```python
from build123d import *

# Parameters (mm, degrees)
SKETCH3_R                = 15
BOSS_EXTRUDE2_DEPTH      = 40
BOSS_EXTRUDE3_DEPTH      = 30
BOSS_EXTRUDE3_DEPTH_BACK = 30
SKETCH4_R                = 10
SKETCH5_OUTSIDE_W        = 57.62
SKETCH5_OUTSIDE_H        = 47.62
SKETCH5_OUTSIDE_R        = 10
SKETCH5_OUTSIDE_R_2      = 6
CUT_EXTRUDE2_DEPTH       = 10


with BuildPart() as part:
    # Sketch3 → Boss-Extrude2 (new body)
    with BuildSketch(Plane.XY):
        Circle(SKETCH3_R)
    extrude(amount=BOSS_EXTRUDE2_DEPTH)

    # Sketch4 → Boss-Extrude3 (add, two sides: drawn at the far end of the back side and taken through both)
    with BuildSketch(Plane(origin=(0, 0, 0), x_dir=(0, 0, -1), z_dir=(1, 0, 0)).offset(-BOSS_EXTRUDE3_DEPTH_BACK)):
        with Locations((-20, 0)):
            Circle(SKETCH4_R)
    extrude(amount=BOSS_EXTRUDE3_DEPTH + BOSS_EXTRUDE3_DEPTH_BACK)

    # Sketch5 outside → Cut-Extrude2 (cut)
    # profile 1 of 2: a face of its own
    with BuildSketch(Plane(origin=(30, 0, 0), x_dir=(0, 0, -1), z_dir=(1, 0, 0))):
        with Locations((-20, 0)):
            Rectangle(SKETCH5_OUTSIDE_W, SKETCH5_OUTSIDE_H)
        with Locations((-20, 0)):
            Circle(SKETCH5_OUTSIDE_R, mode=Mode.SUBTRACT)
    # profile 2 of 2: a face of its own
    with BuildSketch(Plane(origin=(30, 0, 0), x_dir=(0, 0, -1), z_dir=(1, 0, 0))):
        with Locations((-20, 0)):
            Circle(SKETCH5_OUTSIDE_R_2)
    extrude(amount=-CUT_EXTRUDE2_DEPTH, mode=Mode.SUBTRACT)


solid = part.part
```
Input: part model. Units: mm. Frame: model coordinates. A direction names the side the tool comes from. Round coordinates to 2 decimals unless told otherwise and drop trailing zeros. Loops run counter-clockwise (first coordinate to the right, second up) from the corner with the lowest first, then second, coordinate; pieces in that order, holes last. Notation, with made-up numbers: (-5, 41.5) - (9, 41.5) arc R9 cw to (9, 52.5) - close; hole circle Ø8 at (30, -2). An arc over 180 degrees is marked (long way). One line per item, written item: value. Start each with the question number.
(1) Section D-D, the plane x = 17.5. Return loops of the section in (y, z), plus the area to 3 significant figures.
(2) Ray query, line 1 (Y direction, x = 25.75, z = 20); line 2 (X direction, y = 0.5, z = 25.5); line 3 (Y direction, x = -23, z = 20.5). Return the intervals inside material, ascending. Write a range as [from, to].
(3) Contact query for flat-ended pins moving along their axis: P1, Ø8, axis at x = 19, z = 7.5, coming from the -Y side; P2, Ø4, axis at y = -9, z = 4.5, coming from the -X side; P3, Ø6, axis at x = -24, y = 6.5, coming from the -Z side. Output: stop coordinate, or through.
(4) Access query for faces 1 (the cylindrical face through (-11.056, 10.138, 19.72)), 2 (the cylindrical face through (-21, -6, 28)), 3 (the flat face through (20, 0, 20)). Directions: +Z, -Z, +X, -X, +Y, -Y. A direction counts if a zero-diameter tool reaches every point of the face in a straight line with its end or side. Return the directions, or none.
(5) Section C-C, the plane x = 26. Return loops of the section in (y, z).
(6) Draft query along Y for faces 4 (the flat face through (0, 0, 40)), 5 (the cylindrical face through (23, 0, 30)), 6 (the cylindrical face through (25.07, -3.65, 24.76)). Return one class per face: +Y half, -Y half, draft (parallel to the pull), parting line (faces both ways), or undercut.
(7) Section A-A, the plane z = 20. Return loops of the section in (x, y), plus the area to 3 significant figures.
(8) Section B-B, the plane y = 0. Return loops of the section in (x, z), plus the area to 3 significant figures.
Results below:
1. outline: circle Ø20 at (0, 20)
1. area: 314 mm^2
2. line 1: [-10, -6], [6, 10]
2. line 2: [-30, 20]
2. line 3: [-9.99, 9.99]
3. P1: y = -5.27
3. P2: x = -13.27
3. P3: z = 10.63
4. face 1: none
4. face 2: -X
4. face 3: +X
5. outline: circle Ø20 at (0, 20); hole circle Ø12 at (0, 20)
6. face 4: draft
6. face 5: parting line
6. face 6: undercut
7. outline: (-30, -10) - (-11.18, -10) arc R15 ccw to (11.18, -10) - (30, -10) - (30, -6) - (20, -6) - (20, 6) - (30, 6) - (30, 10) - (11.18, 10) arc R15 ccw to (-11.18, 10) - (-30, 10) - close
7. area: 1,230 mm^2
8. outline: (-30, 10) - (-15, 10) - (-15, 0) - (15, 0) - (15, 10) - (30, 10) - (30, 14) - (20, 14) - (20, 26) - (30, 26) - (30, 30) - (15, 30) - (15, 40) - (-15, 40) - (-15, 30) - (-30, 30) - close
8. area: 1,680 mm^2
